Work out the finished part from the listing and answer in its coordinate system (mm). Round coordinates to 2 decimals unless told otherwise and drop trailing zeros. Order: outer loops, then holes, each group sorted by start corner. A loop starts at its lowest first (then second) coordinate and runs counter-clockwise, first axis right, second up. Notation, with made-up numbers: (5.5, -32) - (53.5, -32) arc R4 cw to (53.5, -26) - close; hole circle Ø9 at (70.5, -24.5). An arc over 180 degrees is marked (long way). Put each result on its own line as item: value.
Autodesk Inventor part; units mm, degrees
ref_plane "YZ Plane" through (0, 0, 0) normal (1, 0, 0) x (0, 1, 0)
ref_plane "XZ Plane" through (0, 0, 0) normal (0, 1, 0) x (-1, 0, 0)
ref_plane "XY Plane" through (0, 0, 0) normal (0, 0, 1) x (1, 0, 0)
sketch "스케치1" plane through (0, 0, 0) normal (0, 0, 1) x (1, 0, 0)
  line L0 (-48.1, 15) -> (48.1, 15)
  line L1 (48.1, 15) -> (48.1, -15)
  line L2 (48.1, -15) -> (-48.1, -15)
  line L3 (-48.1, -15) -> (-48.1, 15)
  line L4 (-48.1, 15) -> (48.1, -15) construction
  line L5 (48.1, 15) -> (-48.1, -15) construction
  point P0 (0, 0)
  dimension "d0" = 96.2
  dimension "d1" = 30
extrude "돌출1" add sketch "스케치1" along normal blind 4
sketch "스케치2" plane through (0, 0, 4) normal (0, 0, 1) x (1, 0, 0)
  line L0 (-48.1, 15) -> (-48.1, -15)
  line L1 (-48.1, 0) -> (48.1, 0) construction
  line L2 (48.1, -15) -> (48.1, 15)
  circle A0 centre (-24, 0) radius 1.6
  circle A1 centre (-34, 0) radius 1.6
  circle A2 centre (14, 0) radius 1.6
  circle A3 centre (24, 0) radius 1.6
  circle A4 centre (34, 0) radius 1.6
  circle A5 centre (-14, 0) radius 1.6
  point P0 (0, 0)
  point P1 (0, 0)
  dimension "d5" = 3.2
  dimension "d6" = 3.2
  dimension "d7" = 3.2
  dimension "d8" = 3.2
  dimension "d9" = 14
  dimension "d10" = 10
  dimension "d11" = 3.2
  dimension "d12" = 3.2
  dimension "d13" = 10
  dimension "d14" = 14
  dimension "d15" = 10
  dimension "d16" = 10
extrude "돌출2" cut sketch "스케치2" against normal blind 4
fillet "모깎기1" radius 6 4 edges at (-48.1, 15, 2) (-48.1, -15, 2) (48.1, -15, 2) (48.1, 15, 2)
sketch "스케치3" plane through (0, 0, 4) normal (0, 0, 1) x (1, 0, 0)
  arc A0 (48.1, 9) -> (42.1, 15) centre (42.1, 9) ccw
  line L0 (42.1, 15) -> (-42.1, 15)
  arc A1 (-42.1, 15) -> (-48.1, 9) centre (-42.1, 9) ccw
  line L1 (-48.1, 9) -> (-48.1, -9)
  arc A2 (-48.1, -9) -> (-42.1, -15) centre (-42.1, -9) ccw
  line L2 (-42.1, -15) -> (42.1, -15)
  arc A3 (42.1, -15) -> (48.1, -9) centre (42.1, -9) ccw
  line L3 (48.1, -9) -> (48.1, 9)
  circle A4 centre (-14, 0) radius 1.6
  circle A5 centre (34, 0) radius 1.6
  circle A6 centre (-24, 0) radius 1.6
  circle A7 centre (14, 0) radius 1.6
  circle A8 centre (24, 0) radius 1.6
  circle A9 centre (-34, 0) radius 1.6
  circle A10 centre (-38.1, 10) radius 1.35
  circle A11 centre (-13.1, 10) radius 1.35
  circle A12 centre (-38.1, -10) radius 1.35
  circle A13 centre (-13.1, -10) radius 1.35
  line L4 (0, 0) -> (0, 15)
  line L5 (42.1, 15) -> (-42.1, 15)
  line L6 (48.1, 9) -> (48.1, -9)
  circle A14 centre (38.1, 10) radius 1.35
  circle A15 centre (13.1, 10) radius 1.35
  circle A16 centre (38.1, -10) radius 1.35
  circle A17 centre (13.1, -10) radius 1.35
  dimension "d20" = 2.7
  dimension "d21" = 2.7
  dimension "d22" = 2.7
  dimension "d23" = 2.7
  dimension "d24" = 25
  dimension "d25" = 25
  dimension "d26" = 20
  dimension "d27" = 10
  dimension "d28" = 10
extrude "돌출3" cut sketch "스케치3" against normal blind 4 contours A10 | A11 | A12 | A13 | A14 | A15 | A16 | A17
properties part number "lm가이드가이드" material "알루미늄 6061"
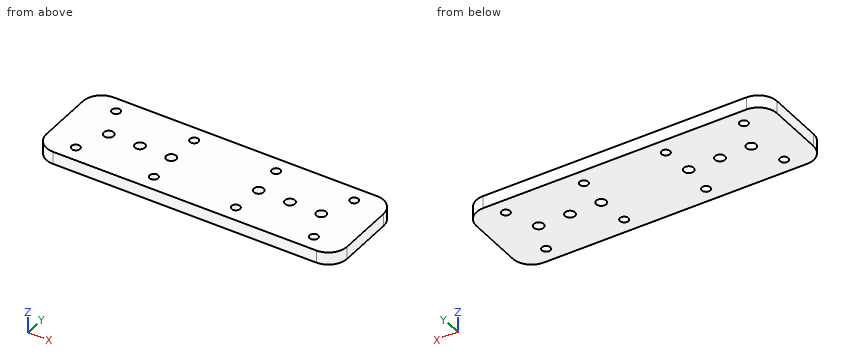
1) A cutting plane is placed at D-D on z = 2.1. Give the number of separate pieces and of enclosed holes in the cut face, then the cut area to 3 significant figures.
Findings below:
separate pieces: 1
enclosed holes: 14
area: 2,760 mm2
2) Straight lines are drawn through the part: L1, parallel to Y at x = -38.1, z = 1.8; L2, parallel to Y at x = 13.1, z = 2.4; L3, parallel to Y at x = -24, z = 1.9. For each, find the intervals that lie inside material, in ascending order. Write a range as from..to.
Findings below:
L1: y = -15..-11.35, -8.65..8.65, 11.35..15
L2: y = -15..-11.35, -8.65..-1.32, 1.32..8.65, 11.35..15
L3: y = -15..-1.6, 1.6..15
3) A cutting plane is placed at B-B on y = 0. Write down the section's boundary in (x, z), then the cut area to 3 significant figures.
Findings below:
outline: (-48.1, 0) - (-35.6, 0) - (-35.6, 4) - (-48.1, 4) - close; (-32.4, 0) - (-25.6, 0) - (-25.6, 4) - (-32.4, 4) - close; (-22.4, 0) - (-15.6, 0) - (-15.6, 4) - (-22.4, 4) - close; (-12.4, 0) - (12.4, 0) - (12.4, 4) - (-12.4, 4) - close; (15.6, 0) - (22.4, 0) - (22.4, 4) - (15.6, 4) - close; (25.6, 0) - (32.4, 0) - (32.4, 4) - (25.6, 4) - close; (35.6, 0) - (48.1, 0) - (48.1, 4) - (35.6, 4) - close
area: 308 mm2
4) A cutting plane is placed at A-A on x = 38.1. Write down the section's boundary in (y, z).
Findings below:
outline: (-15, 0) - (-11.35, 0) - (-11.35, 4) - (-15, 4) - close; (-8.65, 0) - (8.65, 0) - (8.65, 4) - (-8.65, 4) - close; (11.35, 0) - (15, 0) - (15, 4) - (11.35, 4) - close
5) A cutting plane is placed at C-C on x = -24. Write down the section's boundary in (y, z), then the cut area to 3 significant figures.
Findings below:
outline: (-15, 0) - (-1.6, 0) - (-1.6, 4) - (-15, 4) - close; (1.6, 0) - (15, 0) - (15, 4) - (1.6, 4) - close
area: 107 mm2
